Verification items for the finished model (mm, model axes). A direction names the side the tool comes from. Coordinates: 2 decimals unless noted, no trailing zeros. Order: outer loops, then holes, each group sorted by start corner. A loop starts at its lowest first (then second) coordinate and runs counter-clockwise, first axis right, second up. Notation, with made-up numbers: (-17, -8) -> (19, -8) arc R18 ccw to (19, 21) -> close; hole circle Ø7 at (4.25, 27). An arc over 180 degrees is marked (long way). Write each question's results on one line, items separated by ' | '. Start each with the question number.
(1) Go/stop test with flat-tipped pins: pin 1 (13 mm diameter, centred on x = 161.5, z = 12, fed in from +Y); pin 2 (12 mm diameter, centred on x = 88, z = 6.5, fed in from -Y); pin 3 (3 mm diameter, centred on x = -107.95, y = 0, fed in from +Z); pin 4 (1.8 mm diameter, centred on x = 88.9, y = 14.29, fed in from -Z). Record where each tip stops, or that it passes through.
(2) Cross-section at A-A on z = -24. Enter the section's corners in (x, y).
(3) Cross-section at D-D on y = 120.5. Enter the section's corners in (x, z), and give its area (3 significant figures).
(4) Set-up check for faces 1 (the flat face through (-146.05, -22, 1)), 2 (the cylindrical face through (-26.29, 26.69, 0.18)), 3 (the cylindrical face through (64.46, -123.94, -0.89)), 4 (the flat face through (10, 1, 12.7)): record each of +Z, -Z, +X, -X, +Y, -Y from which the full face is reachable in a straight line by a thin tool's end or side.
(5) Cross-section at B-B on x = -92. Enter the section's corners in (y, z), and give its area (3 significant figures).
(6) Draft check along Y on faces 5 (the flat face through (-80, -19.05, 0)), 6 (the flat face through (-133, -44, -63.5)), 7 (the flat face through (165, 6.35, 1)), 8 (the flat face through (94, 19.05, 0)). Enter one of: +Y half, -Y half, draft (parallel to the pull), parting line (faces both ways), or undercut.
(7) Thickness scan on probe 1 along Y at (x, z) = (88, 7); probe 2 along X at (y, z) = (127, 0.5); probe 3 along Y at (x, z) = (-107.95, 2.25). Record the ranges inside material, lowest first. Write a range as [from, to].
(8) Cross-section at C-C on y = -10.5. Enter the section's corners in (x, z) (3 decimals).
```python
from build123d import *

# Parameters (mm, degrees)
SKETCH1_R               = 152.4
SKETCH1_R_2             = 139.7
BOSS_EXTRUDE1_DEPTH     = 63.5
BOSS_EXTRUDE2_DEPTH     = 12.7
CUT_EXTRUDE3_DEPTH      = 225.685936365
CUT_EXTRUDE3_DEPTH_BACK = 225.685936365
SKETCH4_W               = 19.05
SKETCH4_H               = 19.05
SKETCH7_W               = 19.05
SKETCH7_H               = 6.35
CUT_EXTRUDE4_DEPTH      = 229.6
SKETCH8_W               = 17.202693119
SKETCH8_H               = 50.8
CUT_EXTRUDE5_DEPTH      = 251.160988166
SKETCH9_W               = 31.75
SKETCH9_H               = 6.35
BOSS_EXTRUDE3_DEPTH     = 127
SKETCH10_W              = 6.35
SKETCH10_H              = 1.5875
CUT_EXTRUDE6_DEPTH      = 247.262136757
F_4_40_TAPPED_HOLE1_D   = 2.2606
F_6_32_TAPPED_HOLE1_D   = 2.7051
CIRPATTERN1_COUNT       = 4


with BuildPart() as part:
    # Sketch1 → Boss-Extrude1 (new, symmetric)
    with BuildSketch(Plane.XY):
        Circle(SKETCH1_R)
        Circle(SKETCH1_R_2, mode=Mode.SUBTRACT)
    extrude(amount=BOSS_EXTRUDE1_DEPTH, both=True)

    # Sketch2 → Boss-Extrude2 (add, symmetric)
    with BuildSketch(Plane.XY):
        with BuildLine():
            ThreePointArc((-114.3, 19.05), (-127.736482233, 28.655491493), (-132.425396447, 44.492745205))
            Line((-132.425396447, 44.492745205), (-143.350279695, 19.05))
            Line((-143.350279695, 19.05), (-147.191797275, 19.05))
            Line((-147.191797275, 19.05), (-147.191797275, -19.05))
            Line((-147.191797275, -19.05), (-143.95681272, -19.05))
            Line((-143.95681272, -19.05), (-132.439750453, -44.45))
            ThreePointArc((-132.439750453, -44.45), (-127.731621931, -28.635000127), (-114.3, -19.05))
            Line((-114.3, -19.05), (-44.45, -19.05))
            ThreePointArc((-44.45, -19.05), (-26.489487758, -26.489487758), (-19.05, -44.45))
            Line((-19.05, -44.45), (-19.05, -114.3))
            ThreePointArc((-19.05, -114.3), (-28.655491493, -127.736482233), (-44.492745205, -132.425396447))
            Line((-44.492745205, -132.425396447), (-19.05, -143.350279695))
            Line((-19.05, -143.350279695), (-19.05, -143.95681272))
            Line((-19.05, -143.95681272), (19.05, -143.95681272))
            Line((19.05, -143.95681272), (44.45, -132.439750453))
            ThreePointArc((44.45, -132.439750453), (28.635000127, -127.731621931), (19.05, -114.3))
            Line((19.05, -114.3), (19.05, -44.45))
            ThreePointArc((19.05, -44.45), (26.489487758, -26.489487758), (44.45, -19.05))
            Line((44.45, -19.05), (114.3, -19.05))
            ThreePointArc((114.3, -19.05), (127.736482233, -28.655491493), (132.425396447, -44.492745205))
            Line((132.425396447, -44.492745205), (143.350279695, -19.05))
            Line((143.350279695, -19.05), (147.191797275, -19.05))
            Line((147.191797275, -19.05), (147.191797275, 19.05))
            Line((147.191797275, 19.05), (143.95681272, 19.05))
            Line((143.95681272, 19.05), (132.439750453, 44.45))
            ThreePointArc((132.439750453, 44.45), (127.731621931, 28.635000127), (114.3, 19.05))
            Line((114.3, 19.05), (44.45, 19.05))
            ThreePointArc((44.45, 19.05), (26.489487758, 26.489487758), (19.05, 44.45))
            Line((19.05, 44.45), (19.05, 114.3))
            ThreePointArc((19.05, 114.3), (28.655491493, 127.736482233), (44.492745205, 132.425396447))
            Line((44.492745205, 132.425396447), (19.05, 143.350279695))
            Line((19.05, 143.350279695), (19.05, 143.95681272))
            Line((19.05, 143.95681272), (-19.05, 143.95681272))
            Line((-19.05, 143.95681272), (-44.45, 132.439750453))
            ThreePointArc((-44.45, 132.439750453), (-28.635000127, 127.731621931), (-19.05, 114.3))
            Line((-19.05, 114.3), (-19.05, 44.45))
            ThreePointArc((-19.05, 44.45), (-26.489487758, 26.489487758), (-44.45, 19.05))
            Line((-44.45, 19.05), (-114.3, 19.05))
        make_face()
    extrude(amount=BOSS_EXTRUDE2_DEPTH, both=True)

    # Sketch4 → Cut-Extrude3 (cut, two sides: drawn at the far end of the back side and taken through both)
    with BuildSketch(Plane.XY.offset(-CUT_EXTRUDE3_DEPTH_BACK)):
        with Locations((0, -9.525)):
            Rectangle(SKETCH4_W, SKETCH4_H)
    extrude(amount=CUT_EXTRUDE3_DEPTH + CUT_EXTRUDE3_DEPTH_BACK, mode=Mode.SUBTRACT)

    # Sketch7 → Cut-Extrude4 (cut, through all)
    with BuildSketch(Plane.XY.offset(12.7)):
        with Locations((0, 3.175)):
            Rectangle(SKETCH7_W, SKETCH7_H)
    extrude(amount=-CUT_EXTRUDE4_DEPTH, mode=Mode.SUBTRACT)

    # Sketch8 → Cut-Extrude5 (cut, through all)
    with BuildSketch(Plane.XY.offset(63.5)):
        with Locations((-154.65134656, -25.4)):
            Rectangle(SKETCH8_W, SKETCH8_H)
    cut_extrude5 = extrude(amount=-CUT_EXTRUDE5_DEPTH, mode=Mode.SUBTRACT)

    # Mirror1: Cut-Extrude5 across plane
    add(cut_extrude5.mirror(Plane(origin=(0, 0, 0), x_dir=(0, 0, 1), z_dir=(1, 0, 0))), mode=Mode.SUBTRACT)

    # Sketch9 → Boss-Extrude3 (add)
    with BuildSketch(Plane.XY.offset(63.5)):
        with Locations((161.925, 3.175)):
            Rectangle(SKETCH9_W, SKETCH9_H)
    boss_extrude3 = extrude(amount=-BOSS_EXTRUDE3_DEPTH)

    # Mirror2: Boss-Extrude3 across plane
    add(boss_extrude3.mirror(Plane(origin=(0, 0, 0), x_dir=(0, 0, 1), z_dir=(1, 0, 0))))

    # Sketch10 → Cut-Extrude6 (cut, through all)
    with BuildSketch(Plane.XY.offset(12.7)):
        with Locations((-69.85, 18.25625)):
            Rectangle(SKETCH10_W, SKETCH10_H)
    cut_extrude6 = extrude(amount=-CUT_EXTRUDE6_DEPTH, mode=Mode.SUBTRACT)

    # Mirror3: Cut-Extrude6 across plane
    add(cut_extrude6.mirror(Plane(origin=(0, 0, 0), x_dir=(0, 0, 1), z_dir=(1, 0, 0))), mode=Mode.SUBTRACT)

    # #4-40 Tapped Hole1 (through all)
    with Locations(Plane.XY.offset(12.7)):
        with Locations((-14.2875, 63.5), (-6.0325, 63.5), (88.9, 14.2875), (88.9, 6.0325)):
            Hole(F_4_40_TAPPED_HOLE1_D / 2)

    # #6-32 Tapped Hole1 (through all)
    with Locations(Plane.XY.offset(12.7)):
        with Locations((-107.95, 0), (-127, 0)):
            f_6_32_tapped_hole1 = Hole(F_6_32_TAPPED_HOLE1_D / 2)

    # CirPattern1: #6-32 Tapped Hole1 ×4 about axis
    cirpattern1_axis = Axis((0, 0, 0), (0, 0, 1))
    for i in range(1, CIRPATTERN1_COUNT):
        add(f_6_32_tapped_hole1.rotate(cirpattern1_axis, i * 360 / CIRPATTERN1_COUNT), mode=Mode.SUBTRACT)


solid = part.part
```
Results are:
1) pin 1: stops at y = 6.35 | pin 2: stops at y = -128.46 | pin 3: stops at z = 12.7 | pin 4: passes through
2) outline: (-177.8, 0) -> (-146.05, 0) -> (-146.05, -43.53) arc R152.4 ccw to (146.05, -43.53) -> (146.05, 0) -> (177.8, 0) -> (177.8, 6.35) -> (152.27, 6.35) arc R152.4 ccw to (-152.27, 6.35) -> (-177.8, 6.35) -> close; hole circle Ø279.4 at (0, 0)
3) outline: (-93.3, -63.5) -> (-70.68, -63.5) -> (-70.68, 63.5) -> (-93.3, 63.5) -> close; (-21.84, -12.7) -> (21.85, -12.7) -> (21.85, 12.7) -> (-21.84, 12.7) -> close; (70.68, -63.5) -> (93.3, -63.5) -> (93.3, 63.5) -> (70.68, 63.5) -> close | area: 6,860 mm2
4) face 1: +Z, -Z, -X, -Y | face 2: +Z, -Z | face 3: none | face 4: +Z
5) outline: (-121.5, -63.5) -> (-105.13, -63.5) -> (-105.13, 63.5) -> (-121.5, 63.5) -> close; (-19.05, -12.7) -> (19.05, -12.7) -> (19.05, 12.7) -> (-19.05, 12.7) -> close; (105.13, -63.5) -> (121.5, -63.5) -> (121.5, 63.5) -> (105.13, 63.5) -> close | area: 5,130 mm2
6) face 5: undercut | face 6: draft | face 7: +Y half | face 8: undercut
7) probe 1: y = [-124.43, -108.5], [-19.05, 5.35], [6.72, 13.6], [14.97, 19.05], [108.5, 124.43] | probe 2: x = [-84.24, -58.2], [-27.66, -1.35], [1.35, 27.67], [58.2, 84.24] | probe 3: y = [-107.58, -88.67], [-19.05, -1.35], [1.35, 19.05], [88.67, 107.58]
8) outline: (-146.05, -63.5) -> (-139.305, -63.5) -> (-139.305, -12.7) -> (-9.525, -12.7) -> (-9.525, 12.7) -> (-139.305, 12.7) -> (-139.305, 63.5) -> (-146.05, 63.5) -> close; (9.525, -12.7) -> (139.305, -12.7) -> (139.305, -63.5) -> (146.05, -63.5) -> (146.05, 63.5) -> (139.305, 63.5) -> (139.305, 12.7) -> (9.525, 12.7) -> close
